```python
from build123d import *

# Parameters (mm, degrees)
BASPROSKE_W         = 6.35
BASPROSKE_H         = 7.62
TOOTHCUT_DEPTH      = 13.508049408
TEETHCUTS_COUNT     = 10
TEETHCUTS_ANGLE     = 324
BORSKE_R            = 2.38125
BORE_DEPTH          = 50.8000508
BOSS_EXTRUDE1_DEPTH = 6.35


with BuildPart() as part:
    # BasProSke → Base-Revolve (revolve)
    with BuildSketch(Plane(origin=(0, 0, 0), x_dir=(1, 0, 0), z_dir=(0, 1, 0)), mode=Mode.PRIVATE) as base_revolve_sk:
        with Locations((3.175, 3.81)):
            Rectangle(BASPROSKE_W, BASPROSKE_H)
    revolve(base_revolve_sk.sketch.rotate(Axis((-10, 0, 0), (1, 0, 0)), 180), axis=Axis((-10, 0, 0), (1, 0, 0)))

    # TooCutSke → ToothCut (cut, through all)
    with BuildSketch(Plane(origin=(0, 0, 0), x_dir=(0, 0, -1), z_dir=(1, 0, 0))):
        with BuildLine():
            ThreePointArc((0.754581835, 4.715203208), (0, 4.7752), (-0.754581835, 4.715203208))
            ThreePointArc((-0.754581835, 4.715203208), (-1.08060133, 6.254605234), (-2.250824617, 7.306567573))
            ThreePointArc((-2.250824617, 7.306567573), (0, 7.6454), (2.250824617, 7.306567573))
            ThreePointArc((2.250824617, 7.306567573), (1.08060133, 6.254605234), (0.754581835, 4.715203208))
        make_face()
    toothcut = extrude(amount=TOOTHCUT_DEPTH, mode=Mode.SUBTRACT)

    # TeethCuts: ToothCut ×10 about axis
    teethcuts_axis = Axis((-10, 0, 0), (1, 0, 0))
    for i in range(1, TEETHCUTS_COUNT):
        add(toothcut.rotate(teethcuts_axis, i * TEETHCUTS_ANGLE / (TEETHCUTS_COUNT - 1)), mode=Mode.SUBTRACT)

    # BorSke → Bore (cut, symmetric)
    with BuildSketch(Plane(origin=(0, 0, 0), x_dir=(0, 0, -1), z_dir=(1, 0, 0))):
        with Locations(Location((0, 0, 0), (0, 0, 180))):
            Circle(BORSKE_R)
    extrude(amount=BORE_DEPTH, both=True, mode=Mode.SUBTRACT)

    # Sketch1 → Boss-Extrude1 (add)
    with BuildSketch(Plane(origin=(6.35, 0, 0), x_dir=(0, 0, -1), z_dir=(1, 0, 0))):
        with BuildLine():
            Line((-1.680087888, 1.6875), (1.680087888, 1.6875))
            ThreePointArc((1.680087888, 1.6875), (0, 2.38125), (-1.680087888, 1.6875))
        make_face()
        with BuildLine():
            ThreePointArc((-1.6875, 1.680087888), (-2.38125, 0), (-1.6875, -1.680087888))
            Line((-1.6875, -1.680087888), (-1.6875, 1.680087888))
        make_face()
        with BuildLine():
            ThreePointArc((-1.680087888, -1.6875), (0, -2.38125), (1.680087888, -1.6875))
            Line((1.680087888, -1.6875), (-1.680087888, -1.6875))
        make_face()
        with BuildLine():
            Line((1.6875, 1.680087888), (1.6875, -1.680087888))
            ThreePointArc((1.6875, -1.680087888), (2.200989657, -0.908843272), (2.38125, 0))
            ThreePointArc((2.38125, 0), (2.200989657, 0.908843272), (1.6875, 1.680087888))
        make_face()
    extrude(amount=-BOSS_EXTRUDE1_DEPTH)


solid = part.part
```
CAD build for the part. Positions are in the model's coordinates, mm. Coordinates: 2 decimals unless noted, no trailing zeros. Order: outer loops, then holes, each group sorted by start corner. A loop starts at its lowest first (then second) coordinate and runs counter-clockwise, first axis right, second up. Notation, with made-up numbers: M 7,40.25 L 61,40.25 A17 cw 61,62.25 Z; hole C 13,87 d5. An arc over 180 degrees is marked long. Write each question's results on one line, items separated by ' | '. Start each with the question number.
Q1. Cut at D-D (z = -4). List the corners of the cut face in (x, y).
Q2. Flat gauge pins, fed straight in: P1, Ø3, axis at x = 4.5, z = -5.5, coming from the +Y side; P2, Ø2.5, axis at x = 4, z = 0.5, coming from the -Y side; P3, Ø1.5, axis at x = 2, y = 2.5, coming from the -Z side. Where does each tip first touch, or does it go through?
Q3. Cut at B-B (y = -4). List the corners of the cut face in (x, z).
Q4. Cut at C-C (z = -1). List the corners of the cut face in (x, y).
Q5. Drill centre lines: probe 1 along Z at (x, y) = (0.5, 3.5); probe 2 along Z at (x, y) = (3.25, -3.75); probe 3 along Y at (x, z) = (1.25, -5). Where is each one in solid material? Low to high. Write a range as from..to.
Q6. Pull direction Z, two halves, no side cores. Call faces 1 (the flat face through (6.35, 0, 2)), 2 (the cylindrical face through (3.13, 3.87, 2.8)), 3 (the cylindrical face through (3.131, 0.913, 6.242)): +Z half, -Z half, draft (parallel to the pull), parting line (faces both ways), or undercut.
Q7. Cut at A-A (y = -6.5). List the corners of the cut face in (x, z), then the cut area to 3 significant figures.
Found:
1) outline: M 0,-4.09 L 6.35,-4.09 L 6.35,4.09 L 0,4.09 Z
2) P1: y = 4.64 | P2: y = -7.01 | P3: z = -5.84
3) outline: M 0,-6.18 L 6.35,-6.18 L 6.35,-3.89 L 0,-3.89 Z; M 0,-2.61 L 6.35,-2.61 L 6.35,2.61 L 0,2.61 Z; M 0,3.89 L 6.35,3.89 L 6.35,6.18 L 0,6.18 Z
4) outline: M 0,-6.1 L 6.35,-6.1 L 6.35,-1.69 L 0,-1.69 Z; M 0,1.69 L 6.35,1.69 L 6.35,6.1 L 0,6.1 Z
5) probe 1: -5.99..-3.46, -3.25..3.25, 3.46..5.99 | probe 2: -6.1..-3.65, -2.96..2.96, 3.65..6.1 | probe 3: -4.58..-2.46, -0.85..0.85, 2.46..4.58
6) face 1: draft | face 2: undercut | face 3: undercut
7) outline: M 0,-2.76 L 6.35,-2.76 L 6.35,-1.24 L 0,-1.24 Z; M 0,1.24 L 6.35,1.24 L 6.35,2.76 L 0,2.76 Z | area: 19.3 mm²
